```python
from build123d import *

# Parameters (mm, degrees)
SKETCH1_R           = 4.7625
BOSS_EXTRUDE1_DEPTH = 196.25
CUT_EXTRUDE1_DEPTH  = 18.41
SKETCH3_R           = 4.7625
SKETCH3_R_2         = 4
CUT_EXTRUDE2_DEPTH  = 43.57
CUT_EXTRUDE3_DEPTH  = 15.5


with BuildPart() as part:
    # Sketch1 → Boss-Extrude1 (new body)
    with BuildSketch(Plane.XY):
        Circle(SKETCH1_R)
    extrude(amount=BOSS_EXTRUDE1_DEPTH)

    # Sketch2 → Cut-Extrude1 (cut)
    with BuildSketch(Plane.XY.offset(196.25)):
        Polygon((-36.061047486, 0), (-4.7625, 0), (4.7625, 0), (36.061047486, 0), (36.061047486, 62.597094971), (-36.061047486, 62.597094971), align=None)
    extrude(amount=-CUT_EXTRUDE1_DEPTH, mode=Mode.SUBTRACT)

    # Sketch3 → Cut-Extrude2 (cut)
    with BuildSketch(Plane(origin=(0, 0, 0), x_dir=(-1, 0, 0), z_dir=(0, 0, -1))):
        Circle(SKETCH3_R)
        Circle(SKETCH3_R_2, mode=Mode.SUBTRACT)
    extrude(amount=-CUT_EXTRUDE2_DEPTH, mode=Mode.SUBTRACT)

    # Sketch4 → Cut-Extrude3 (cut)
    with BuildSketch(Plane(origin=(0, 0, 0), x_dir=(-1, 0, 0), z_dir=(0, 0, -1))):
        Polygon((-33.946208913, 0), (-4, 0), (4, 0), (33.946208913, 0), (33.946208913, 59.892417826), (-33.946208913, 59.892417826), align=None)
    extrude(amount=-CUT_EXTRUDE3_DEPTH, mode=Mode.SUBTRACT)


solid = part.part
```
Could you check a few things on this model? Use its own coordinates, in mm. A direction names the side the tool comes from. Round coordinates to 2 decimals unless told otherwise and drop trailing zeros. Write each loop counter-clockwise with the first axis right and the second up, starting at its lowest first coordinate (ties: lowest second). Pieces come first, ordered by that corner, then holes. Notation, with made-up numbers: M -2.5,-33.75 L 6.5,-33.75 A20 cw 6.5,-16.75 Z; hole C 16.5,43 d2. An arc over 180 degrees is marked long. Write each question's results on one line, items separated by ' | '. Start each with the question number.
1. Imagine slicing it at B-B on z = 163.5. List the corners of the cut face in (x, y) for me (1 decimal).
2. I need wall thicknesses on L1, parallel to Z at x = 0, y = 1.5; L2, parallel to X at y = 0.5, z = 163; L3, parallel to Y at x = -1, z = 150. Which ranges of each line are inside material? Lowest first, please. Write a range as from..to.
3. Imagine slicing it at A-A on x = 0. List the corners of the cut face in (y, z) for me.
4. On a 3-axis mill with a long thin cutter (end or side, diameter ignored), from which of +Z, -Z, +X, -X, +Y, -Y can I reach the whole of each face in a straight line? I mean faces 1 (the face through (0.867, -3.905, 26.321)), 2 (the face through (0, 0, 187)), 3 (the face through (-1.03, -4.65, 118.84)), 4 (the face through (0, -2, 0)), 5 (the face through (0, 2, 15.5)). Say none if no direction works.
5. I'm going to push flat-ended pins straight in: pin 1 Ø1.2 at (x, y) = (1.5, 2) entering from -Z; pin 2 Ø2 at (y, z) = (1.5, 106) entering from -X; pin 3 Ø5 at (y, z) = (4, 102) entering from +X. Where does each tip first touch, or does it pass through?
6. Imagine slicing it at C-C on y = 1.5. List the corners of the cut face in (x, z) for me, and give its area (3 significant figures).
Result sheet:
1) outline: C 0,0 d9.5
2) L1: z = 15.5..177.84 | L2: x = -4.74..4.74 | L3: y = -4.66..4.66
3) outline: M -4.76,43.57 L -4,43.57 L -4,0 L 0,0 L 0,15.5 L 4,15.5 L 4,43.57 L 4.76,43.57 L 4.76,177.84 L 0,177.84 L 0,196.25 L -4.76,196.25 Z
4) face 1: -Z | face 2: +Z, +X, -X, +Y | face 3: +Z, -Z | face 4: -Z, +X, -X, +Y, -Y | face 5: -Z, +X, -X, +Y
5) pin 1: stops at z = 15.5 | pin 2: stops at x = -4.74 | pin 3: stops at x = 4.52
6) outline: M -4.52,43.57 L -3.71,43.57 L -3.71,15.5 L 3.71,15.5 L 3.71,43.57 L 4.52,43.57 L 4.52,177.84 L -4.52,177.84 Z | area: 1,420 mm^2
